```python
from build123d import *

# Parameters (mm, degrees)
SKETCH1_W           = 138
SKETCH1_H           = 45
SKETCH1_R           = 1.4
BOSS_EXTRUDE1_DEPTH = 1.5
SKETCH2_R           = 1.65
CUT_EXTRUDE1_DEPTH  = 73.591321795
FILLET1_R           = 2


with BuildPart() as part:
    # Sketch1 → Boss-Extrude1 (new body)
    with BuildSketch(Plane(origin=(0, 0, 0), x_dir=(1, 0, 0), z_dir=(0, 1, 0))):
        Rectangle(SKETCH1_W, SKETCH1_H)
        with Locations(Location((-29, 0, 0), (0, 0, 270))):
            Circle(SKETCH1_R, mode=Mode.SUBTRACT)
        with Locations(Location((29, 0, 0), (0, 0, 270))):
            Circle(SKETCH1_R, mode=Mode.SUBTRACT)
    extrude(amount=BOSS_EXTRUDE1_DEPTH)

    # Sketch2 → Cut-Extrude1 (cut, through all)
    with BuildSketch(Plane(origin=(0, 1.5, 0), x_dir=(1, 0, 0), z_dir=(0, 1, 0))):
        with Locations(Location((-65, 18.5, 0), (0, 0, 270))):
            Circle(SKETCH2_R)
        with Locations(Location((-65, -18.5, 0), (0, 0, 270))):
            Circle(SKETCH2_R)
        with Locations(Location((65, 18.5, 0), (0, 0, 270))):
            Circle(SKETCH2_R)
        with Locations(Location((65, -18.5, 0), (0, 0, 270))):
            Circle(SKETCH2_R)
    extrude(amount=-CUT_EXTRUDE1_DEPTH, mode=Mode.SUBTRACT)

    # Fillet1
    fillet1_edges = [part.edges().sort_by_distance(p)[0] for p in [
        (-69, 0.75, -22.5),
        (69, 0.75, -22.5),
        (69, 0.75, 22.5),
        (-69, 0.75, 22.5),
    ]]
    fillet(fillet1_edges, radius=FILLET1_R)


solid = part.part
```
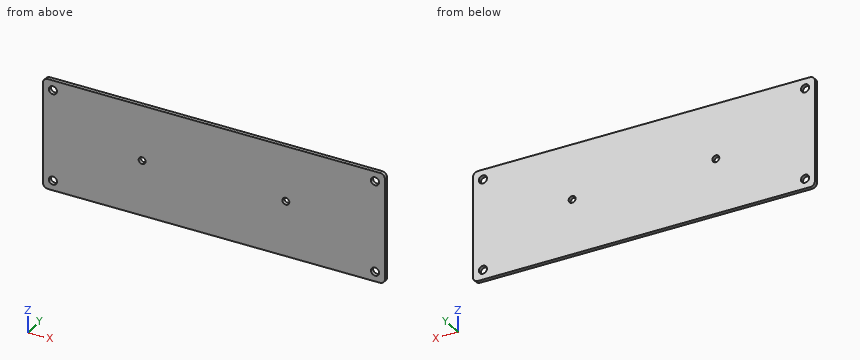
Read the model definition and answer for the solid it produces. Units are mm, in the model's axes. Give positions to 0.01 mm unless a question says otherwise; leave off trailing zeros. Order: outer loops, then holes, each group sorted by start corner. A loop starts at its lowest first (then second) coordinate and runs counter-clockwise, first axis right, second up.
(1) Find section A-A (x = -65). Give the vertices of the cut face in (y, z), plus the area to 3 significant figures.
(2) Find section B-B (z = 18.5). Give the vertices of the cut face in (x, y).
(3) Straight lines are drawn through the part: L1, parallel to Z at x = -65, y = 0.8; L2, parallel to X at y = 0.4, z = 18.5; L3, parallel to X at y = 0.8, z = 0. For each, find the intervals that lie inside material, in ascending order.
Result sheet:
1. outline: (0, -22.5) - (1.5, -22.5) - (1.5, -20.15) - (0, -20.15) - close; (0, -16.85) - (1.5, -16.85) - (1.5, 16.85) - (0, 16.85) - close; (0, 20.15) - (1.5, 20.15) - (1.5, 22.5) - (0, 22.5) - close
1. area: 57.6 mm2
2. outline: (-69, 0) - (-66.65, 0) - (-66.65, 1.5) - (-69, 1.5) - close; (-63.35, 0) - (63.35, 0) - (63.35, 1.5) - (-63.35, 1.5) - close; (66.65, 0) - (69, 0) - (69, 1.5) - (66.65, 1.5) - close
3. L1: z = -22.5 to -20.15, -16.85 to 16.85, 20.15 to 22.5
3. L2: x = -69 to -66.65, -63.35 to 63.35, 66.65 to 69
3. L3: x = -69 to -30.4, -27.6 to 27.6, 30.4 to 69
